from build123d import *

# Parameters (mm, degrees)
CROQUIS1_R                 = 60
CROQUIS1_R_2               = 18.75
CROQUIS1_R_3               = 4
SALIENTE_EXTRUIR1_DEPTH    = 10
CROQUIS2_R                 = 40
CROQUIS2_R_2               = 18.75
SALIENTE_EXTRUIR2_DEPTH    = 50
CHAFL_N2_SIZE              = 0.5
REDONDEO1_R                = 0.5
CROQUIS3_R                 = 4.7625
CORTAR_EXTRUIR1_DEPTH      = 61
CORTAR_EXTRUIR1_DEPTH_BACK = 61
CHAFL_N3_SIZE              = 0.5
REDONDEO3_R                = 0.5


with BuildPart() as part:
    # Croquis1 → Saliente-Extruir1 (new body)
    with BuildSketch(Plane(origin=(0, 0, 0), x_dir=(1, 0, 0), z_dir=(0, 1, 0))):
        Circle(CROQUIS1_R)
        Circle(CROQUIS1_R_2, mode=Mode.SUBTRACT)
        with Locations((25, -43.301270189)):
            Circle(CROQUIS1_R_3, mode=Mode.SUBTRACT)
        with Locations((-25, -43.301270189)):
            Circle(CROQUIS1_R_3, mode=Mode.SUBTRACT)
        with Locations((-50, 0)):
            Circle(CROQUIS1_R_3, mode=Mode.SUBTRACT)
        with Locations((-25, 43.301270189)):
            Circle(CROQUIS1_R_3, mode=Mode.SUBTRACT)
        with Locations((25, 43.301270189)):
            Circle(CROQUIS1_R_3, mode=Mode.SUBTRACT)
        with Locations((50, 0)):
            Circle(CROQUIS1_R_3, mode=Mode.SUBTRACT)
    saliente_extruir1 = extrude(amount=SALIENTE_EXTRUIR1_DEPTH)

    # Croquis2 → Saliente-Extruir2 (add)
    with BuildSketch(Plane(origin=(0, 10, 0), x_dir=(1, 0, 0), z_dir=(0, 1, 0))):
        Circle(CROQUIS2_R)
        Circle(CROQUIS2_R_2, mode=Mode.SUBTRACT)
    extrude(amount=SALIENTE_EXTRUIR2_DEPTH)

    # Chaflán2
    chafl_n2_edges = [part.edges().sort_by_distance(p)[0] for p in [
        (-60, 0, 0),
        (-60, 10, 0),
    ]]
    chamfer(chafl_n2_edges, length=CHAFL_N2_SIZE)

    # Redondeo1
    redondeo1_edges = [part.edges().sort_by_distance(p)[0] for p in [
        (-40, 10, 0),
    ]]
    fillet(redondeo1_edges, radius=REDONDEO1_R)

    # Croquis3 → Cortar-Extruir1 (cut, two sides)
    with BuildSketch(Plane(origin=(0, 0, 0), x_dir=(0, 0, -1), z_dir=(1, 0, 0))) as cortar_extruir1_sk:
        with Locations((0, 35)):
            Circle(CROQUIS3_R)
    extrude(amount=CORTAR_EXTRUIR1_DEPTH, mode=Mode.SUBTRACT)
    extrude(cortar_extruir1_sk.sketch, amount=-CORTAR_EXTRUIR1_DEPTH_BACK, mode=Mode.SUBTRACT)

    # Simetría1: Saliente-Extruir1 across plane
    add(saliente_extruir1.mirror(Plane.ZX.offset(35)))

    # Chaflán3
    chafl_n3_edges = [part.edges().sort_by_distance(p)[0] for p in [
        (-60, 60, 0),
        (-60, 70, 0),
    ]]
    chamfer(chafl_n3_edges, length=CHAFL_N3_SIZE)

    # Redondeo3
    redondeo3_edges = [part.edges().sort_by_distance(p)[0] for p in [
        (-40, 60, 0),
    ]]
    fillet(redondeo3_edges, radius=REDONDEO3_R)


solid = part.part
The listing builds one solid part. Answer for the finished solid, in the listing's coordinates (mm). Round coordinates to 2 decimals unless told otherwise and drop trailing zeros. Order: outer loops, then holes, each group sorted by start corner. A loop starts at its lowest first (then second) coordinate and runs counter-clockwise, first axis right, second up. Notation, with made-up numbers: (56, -6.5) -> (75, -6.5) arc R33 cw to (75, 25.5) -> close; hole circle Ø7 at (41.5, 12.25). An arc over 180 degrees is marked (long way). One line per item, written item: value.
Item 1: Find section B-B, the plane y = 38. Give the vertices of the cut face in (x, z), then the cut area to 3 significant figures.
Taken from the geometry:
outline: (-39.83, -3.7) arc R40 ccw to (39.83, -3.7) -> (18.38, -3.7) arc R18.75 cw to (-18.38, -3.7) -> close; (-39.83, 3.7) -> (-18.38, 3.7) arc R18.75 cw to (18.38, 3.7) -> (39.83, 3.7) arc R40 ccw to start
area: 3,610 mm2
Item 2: Find section C-C, the plane z = 0. State how many separate pieces and enclosed holes the cut face has, then the cut area to 3 significant figures.
Taken from the geometry:
separate pieces: 8
enclosed holes: 0
area: 3,050 mm2
Item 3: Find section A-A, the plane x = 0. Give the vertices of the cut face in (y, z).
Taken from the geometry:
outline: (0, -59.5) -> (0.5, -60) -> (9.5, -60) -> (10, -59.5) -> (10, -40.5) arc R0.5 cw to (10.5, -40) -> (59.5, -40) arc R0.5 cw to (60, -40.5) -> (60, -59.5) -> (60.5, -60) -> (69.5, -60) -> (70, -59.5) -> (70, -18.75) -> (0, -18.75) -> close; (0, 18.75) -> (70, 18.75) -> (70, 59.5) -> (69.5, 60) -> (60.5, 60) -> (60, 59.5) -> (60, 40.5) arc R0.5 cw to (59.5, 40) -> (10.5, 40) arc R0.5 cw to (10, 40.5) -> (10, 59.5) -> (9.5, 60) -> (0.5, 60) -> (0, 59.5) -> close
Item 4: Given P1, Ø1, axis at x = 1, y = 44.5, coming from the +Z side; P2, Ø4, axis at y = 17, z = 27, coming from the -X side (3 decimals); P3, Ø3, axis at x = -8.5, y = 20.5, coming from the +Z side, each flat-ended and moving along its own axis, determine where each tip first touches the part or whether it passes through.
Taken from the geometry:
P1: stops at z = 40
P2: stops at x = -31.225
P3: stops at z = 39.38
Item 5: For a pull along X with two mould halves and no side action, classify faces 1 (the cylindrical face through (-59.94, 65.06, -2.64)), 2 (the cylindrical face through (17.884, 35.49, -5.632)), 3 (the flat face through (-14, 0, -14)) as released by +X, released by -X, zero draft, split by the parting line, or undercut.
Taken from the geometry:
face 1: split by the parting line
face 2: undercut
face 3: zero draft
Item 6: Find section D-D, the plane y = 46. Give the vertices of the cut face in (x, z), then the cut area to 3 significant figures.
Taken from the geometry:
outline: circle Ø80 at (0, 0); hole circle Ø37.5 at (0, 0)
area: 3,920 mm2
Item 7: Straight lines are drawn through the part: L1, parallel to Y at x = -36.5, z = -29.5; L2, parallel to Z at x = 25, y = 67; L3, parallel to Z at x = 1, y = 54. For each, find the intervals that lie inside material, in ascending order.
Taken from the geometry:
L1: y = 0 to 10, 60 to 70
L2: z = -54.54 to -47.3, -39.3 to 39.3, 47.3 to 54.54
L3: z = -39.99 to -18.72, 18.72 to 39.99
